Source: three-view drawing plus pictorial views. Frame: mm from the lowest corner of the part. Coordinates: 2 decimals unless noted, no trailing zeros. Order: outer loops, then holes, each group sorted by start corner. A loop starts at its lowest first (then second) coordinate and runs counter-clockwise, first axis right, second up. Notation, with made-up numbers: M -3,50.5 L 55,50.5 A13 cw 55,73.5 Z; hole C 27.25,-25.75 d3. An arc over 180 degrees is marked long. Write item = value, one per line. Start each with the question number.
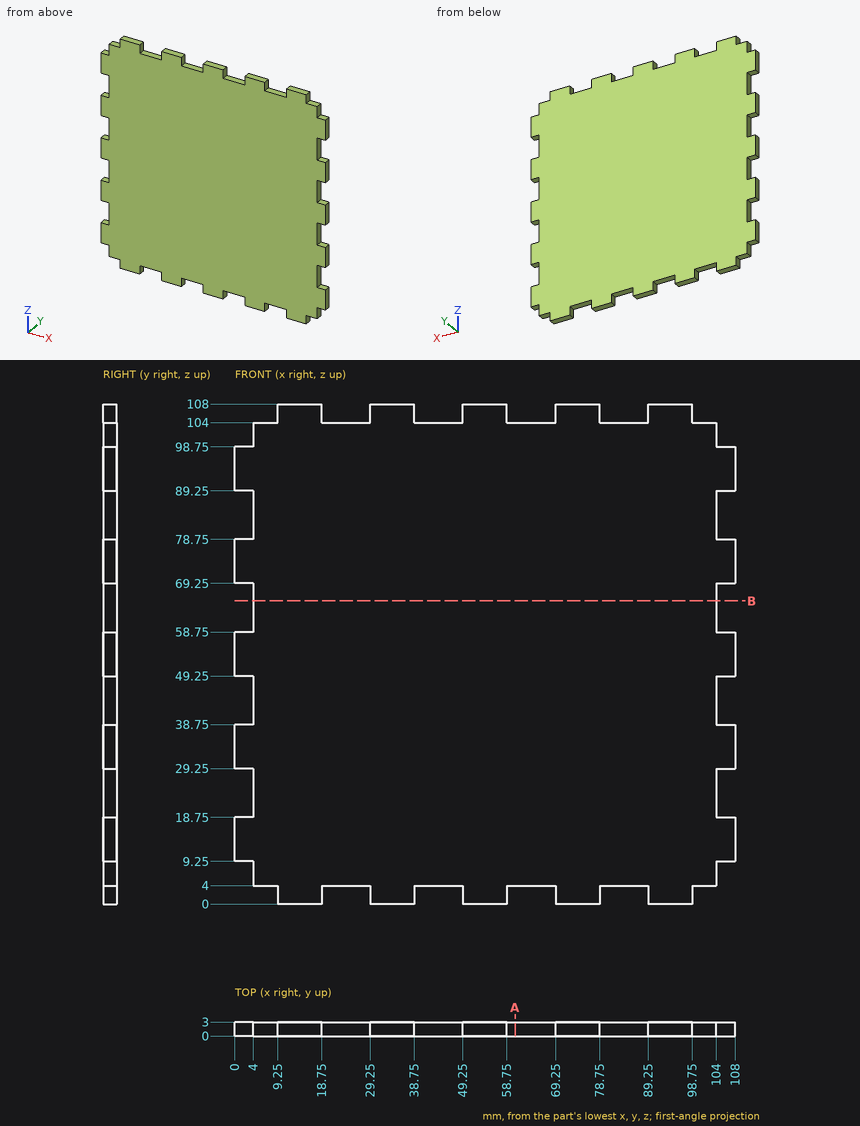
Item 1: Section query B-B on z = 65.5. Output: boundary loops of the cut face in (x, y).
Item 2: Material intervals for probe 1 along X at (y, z) = (0.9, 45.5), sorted ascending. Write a range as [from, to].
Item 3: First-contact query: pin 1 (0.9 mm diameter, centred on y = 2, z = 2, fed in from -X); pin 2 (0.9 mm diameter, centred on y = 1.5, z = 2, fed in from +X); pin 3 (1.5 mm diameter, centred on y = 2, z = 65.5, fed in from +X). Flat tips, straight axial feed; report the tip coordinate or a pass-through.
Item 4: Section query A-A on x = 60.5. Output: boundary loops of the cut face in (y, z), and give its area (3 significant figures).
Ans:
q1.outline = M 4,0 L 104,0 L 104,3 L 4,3 Z
q2.probe_1 = [4, 104]
q3.pin_1 = 9.25
q3.pin_2 = 98.75
q3.pin_3 = 104
q4.outline = M 0,4 L 3,4 L 3,104 L 0,104 Z
q4.area = 300 mm^2
